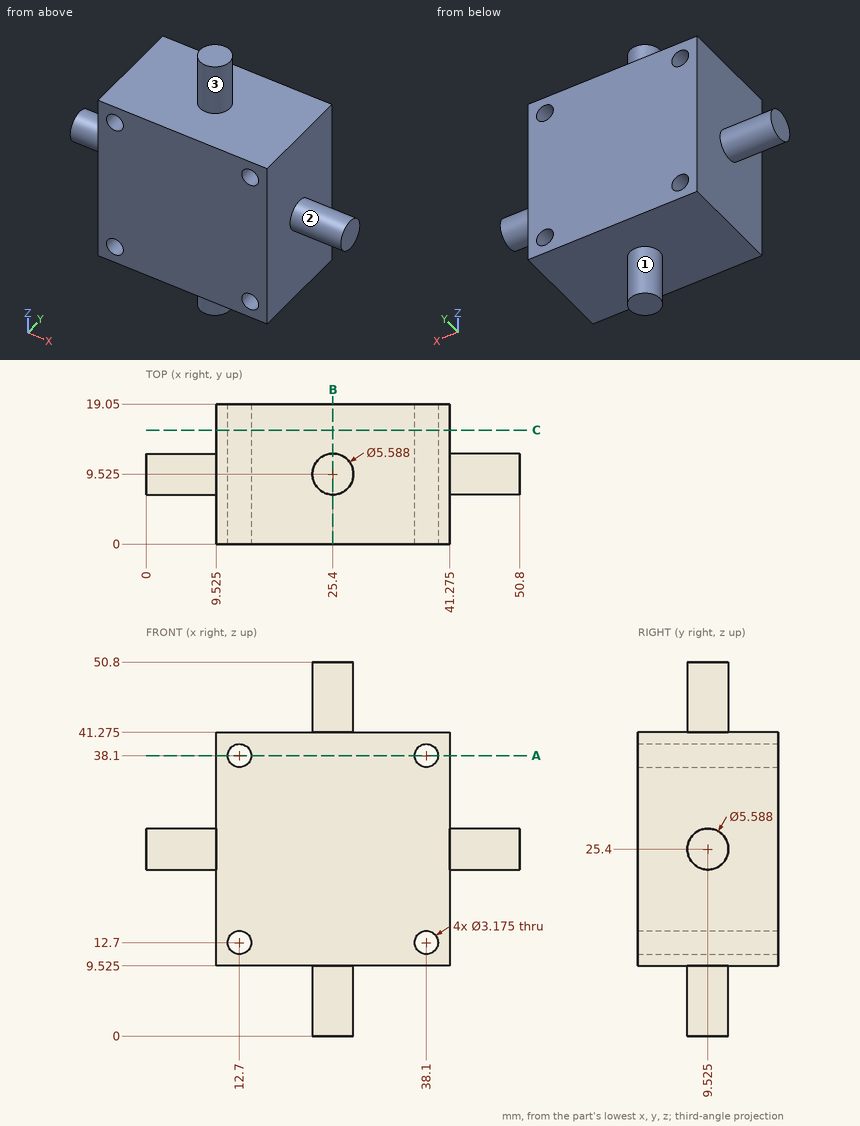
Study the drawing (mm; zero at the part's minimum x, y, z) and answer. A direction names the side the tool comes from. Give positions to 0.01 mm unless a question says otherwise; leave off trailing zeros. Loops run counter-clockwise (first coordinate to the right, second up) from the corner with the lowest first, then second, coordinate; pieces in that order, holes last. Notation, with made-up numbers: M 0,86.25 L 59,86.25 A13 cw 59,107.25 Z; hole C 14,-10.75 d9. An arc over 180 degrees is marked long. One line per item, written item: value. Start each with the question number.
1. Find the intervals of material crossed by probe 1 along X at (y, z) = (6.25, 38.1) (1 decimal); probe 2 along Z at (x, y) = (18, 8.25) (3 decimals), in increasing order.
2. Find section C-C (y = 15.5). Give the vertices of the cut face in (x, z) (1 decimal), and give its area (3 significant figures).
3. Find section B-B (x = 25.4). Give the vertices of the cut face in (y, z) (3 decimals).
4. Each of these flat-tipped pins is pushed along its axis until it touches: P1, Ø3, axis at x = 12.7, z = 38.1, coming from the +Y side; P2, Ø5, axis at y = 15, z = 22, coming from the +X side (3 decimals); P3, Ø5.5, axis at y = 9.5, z = 19.5, coming from the -X side (3 decimals); P4, Ø2, axis at x = 11, y = 2.5, coming from the +Z side (3 decimals). Where does it stop, or does it pass through?
5. Find section A-A (z = 38.1). State how many separate pieces and enclosed holes the cut face has, and give its area (3 significant figures).
6. Which of the six approach directions +Z, -Z, +X, -X, +Y, -Y give full straight-line access (tool end or side, diameter ignored) to the marked faces 1, 2 and 3?
Reported:
1. probe 1: x = 9.5 to 11.1, 14.3 to 36.5, 39.7 to 41.3
1. probe 2: z = 9.525 to 41.275
2. outline: M 9.5,9.5 L 41.3,9.5 L 41.3,41.3 L 9.5,41.3 Z; hole C 12.7,12.7 d3.2; hole C 12.7,38.1 d3.2; hole C 38.1,12.7 d3.2; hole C 38.1,38.1 d3.2
2. area: 976 mm²
3. outline: M 0,9.525 L 6.731,9.525 L 6.731,0 L 12.319,0 L 12.319,9.525 L 19.05,9.525 L 19.05,41.275 L 12.319,41.275 L 12.319,50.8 L 6.731,50.8 L 6.731,41.275 L 0,41.275 Z
4. P1: passes through
4. P2: stops at x = 41.275
4. P3: stops at x = 9.525
4. P4: stops at z = 41.275
5. separate pieces: 3
5. enclosed holes: 0
5. area: 484 mm²
6. face 1: -Z
6. face 2: +X
6. face 3: +Z
